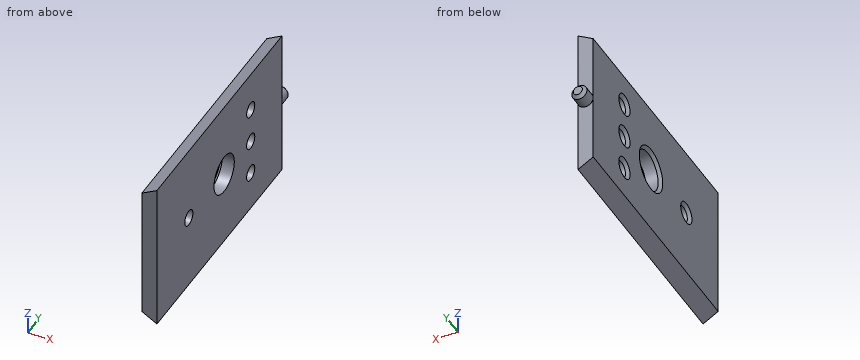
Autodesk Inventor part; units mm, degrees
ref_plane "YZ Plane" through (0, 0, 0) normal (1, 0, 0) x (0, 1, 0)
ref_plane "XZ Plane" through (0, 0, 0) normal (0, 1, 0) x (-1, 0, 0)
ref_plane "XY Plane" through (0, 0, 0) normal (0, 0, 1) x (1, 0, 0)
sketch "스케치2" plane through (0, 0, 0) normal (0, 1, 0) x (-1, 0, 0)
  line L0 (0, 45) -> (38.9711, 22.5)
  line L1 (38.9711, 22.5) -> (38.9711, -22.5)
  line L2 (38.9711, -22.5) -> (0, -45)
  line L3 (0, -45) -> (-38.9711, -22.5)
  line L4 (-38.9711, -22.5) -> (-38.9711, 22.5)
  line L5 (-38.9711, 22.5) -> (0, 45)
  line L6 (0, 50.7735) -> (43.9711, 25.3868)
  line L7 (43.9711, 25.3868) -> (43.9711, -25.3868)
  line L8 (43.9711, -25.3868) -> (0, -50.7735)
  line L9 (0, -50.7735) -> (-43.9711, -25.3868)
  line L10 (-43.9711, -25.3868) -> (-43.9711, 25.3868)
  line L11 (-43.9711, 25.3868) -> (0, 50.7735)
  line L12 (-43.9711, 25.3868) -> (-38.9711, 22.5)
  line L13 (-38.9711, -22.5) -> (-43.9711, -25.3868)
  point P0 (0, 0)
  point P1 (0, 0)
  dimension "d0" = 45
  dimension "d1" = 5
extrude "돌출1" add sketch "스케치2" along normal blind 80 contours L4 L13 L10 L12
sketch "스케치3" plane through (38.9711, 0, -22.5) normal (-1, 0, 0) x (0, 0, 1)
  line L0 (0, 0) -> (45, 0) construction
  circle A0 centre (22.5, 20.4) radius 2.6
  point P0 (22.5, 0)
  point P1 (22.5, 0)
  dimension "d4" = 5.2
  dimension "d5" = 20.4
extrude "돌출2" cut sketch "스케치3" against normal through all
sketch "스케치4" plane through (0, 80, 0) normal (0, 1, 0) x (1, 0, 0)
  line L0 (38.9711, 22.5) -> (38.9711, -22.5) construction
  circle A0 centre (41.4711, 0) radius 2.5
  point P0 (0, 0)
  dimension "d8" = 5
extrude "돌출3" add sketch "스케치4" along normal blind 5
sketch "스케치5" plane through (43.9711, 0, 25.3868) normal (1, 0, 0) x (0, 0, -1)
  line L0 (50.7735, 0) -> (50.7735, 80) construction
  line L1 (25.3868, 80) -> (50.7735, 80) construction
  line L2 (0, 0) -> (0, 80) construction
  circle A0 centre (25.3868, 60) radius 2.6
  circle A1 centre (13.3868, 60) radius 2.6
  circle A2 centre (37.3868, 60) radius 2.6
  line L3 (0, 60) -> (50.7735, 60)
  point P0 (25.3868, 0)
  dimension "d11" = 20
  dimension "d12" = 0
  dimension "d13" = 0
  dimension "d14" = 0
  dimension "d15" = 12
  dimension "d16" = 12
  dimension "d17" = 5.2
  dimension "d18" = 5.2
  dimension "d19" = 5.2
extrude "돌출4" cut sketch "스케치5" against normal through all
sketch "스케치6" plane through (43.9711, 0, 25.3868) normal (1, 0, 0) x (0, 0, -1)
  line L0 (0, 0) -> (50.7735, 0) construction
  circle A0 centre (25.3868, 43) radius 6.5
  point P0 (25.3868, 0)
  dimension "d22" = 13
  dimension "d23" = 43
extrude "돌출5" cut sketch "스케치6" against normal through all
chamfer "모따기1" distance 1 angle 45 6 edges at (38.9711, 85, 0) (38.9711, 60, -9.4) (38.9711, 60, 2.6) (38.9711, 60, 14.6) (38.9711, 43, 6.5) (38.9711, 20.4, -2.6)
properties part number "col_face"
Work out the finished part from the listing and answer in its coordinate system (mm). Give positions to 0.01 mm unless a question says otherwise; leave off trailing zeros. Loops run counter-clockwise (first coordinate to the right, second up) from the corner with the lowest first, then second, coordinate; pieces in that order, holes last. Notation, with made-up numbers: (45.5, 23.5) -> (62.5, 23.5) arc R11 cw to (62.5, 35.5) -> close; hole circle Ø7 at (-1.75, 58.25). An arc over 180 degrees is marked (long way). Use a Markdown table: item, result. Add a question column.
1) Each of these flat-tipped pins is pushed along its axis until it touches: P1, Ø3, axis at y = 60, z = 0, coming from the -X side; P2, Ø7, axis at y = 60, z = 12, coming from the -X side; P3, Ø1.5, axis at x = 40, z = -19.5, coming from the +Y side. Where does it stop, or does it pass through?
2) Consider line 1 along Y through (x, z) = (41.55, 0); line 2 along Y through (x, z) = (43.15, -12); line 3 along Z through (x, y) = (41.7, 60). Determine where each line is inside the solid, lowest interval first.
3) The part is cut by section B-B, the plane y = 20.4. Determine the outline of the cut face in (x, z), plus the area to 3 significant figures.
4) The part is cut by section A-A, the plane z = 12. Determine the outline of the cut face in (x, y).
5) The part is cut by section C-C, the plane y = 70.5. Determine the outline of the cut face in (x, z).
6) The part is cut by section D-D, the plane x = 42.05. Count the separate pieces of the cut face and the enclosed holes in it, plus the area to 3 significant figures.
Reported:
| question | item | result |
|---|---|---|
| 1 | P1 | passes through |
| 1 | P2 | stops at x = 39.07 |
| 1 | P3 | stops at y = 80 |
| 2 | line 1 | y = 0 to 17.8, 23 to 36.5, 49.5 to 57.4, 62.6 to 85 |
| 2 | line 2 | y = 0 to 57.4, 62.6 to 80 |
| 2 | line 3 | z = -24.08 to -14.6, -9.4 to -2.6, 2.6 to 9.4, 14.6 to 24.08 |
| 3 | outline | (38.97, -22.5) -> (43.97, -25.39) -> (43.97, -2.6) -> (39.97, -2.6) -> (38.97, -3.6) -> close; (38.97, 3.6) -> (39.97, 2.6) -> (43.97, 2.6) -> (43.97, 25.39) -> (38.97, 22.5) -> close |
| 3 | area | 212 mm^2 |
| 4 | outline | (38.97, 0) -> (43.97, 0) -> (43.97, 57.4) -> (39.97, 57.4) -> (38.97, 56.4) -> close; (38.97, 63.6) -> (39.97, 62.6) -> (43.97, 62.6) -> (43.97, 80) -> (38.97, 80) -> close |
| 5 | outline | (38.97, -22.5) -> (43.97, -25.39) -> (43.97, 25.39) -> (38.97, 22.5) -> close |
| 6 | separate pieces | 1 |
| 6 | enclosed holes | 5 |
| 6 | area | 3,690 mm^2 |
